The drawing under review shows one solid part. Ordinate dimensions are in mm from its lowest x, y, z. A direction names the side the tool comes from. Round coordinates to 2 decimals unless told otherwise and drop trailing zeros. Order: outer loops, then holes, each group sorted by start corner. A loop starts at its lowest first (then second) coordinate and runs counter-clockwise, first axis right, second up. Notation, with made-up numbers: M -14.5,3.25 L 41.5,3.25 A25 ccw 41.5,39.25 Z; hole C 32.25,-37 d11. An arc over 180 degrees is marked long. Answer as a JSON object with one key per item and string values.
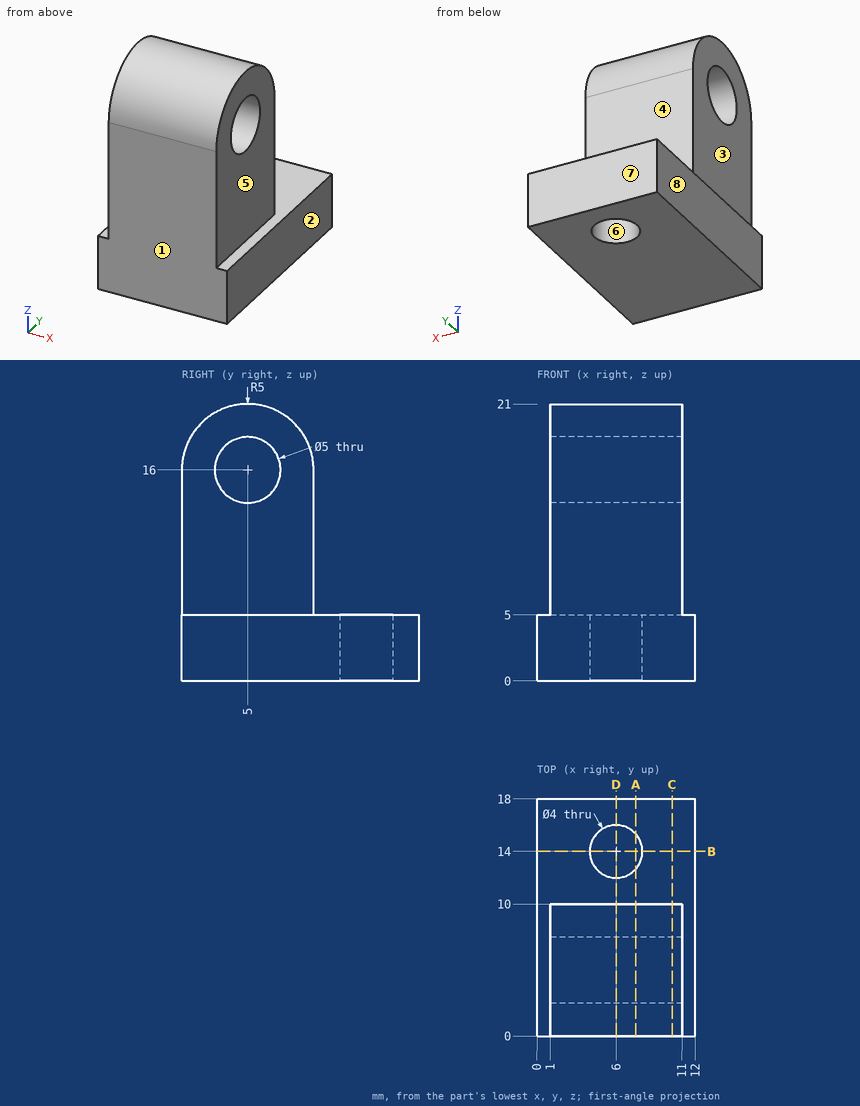
1) Add section D-D on x = 6. State the section outline as (y, z) points, and give its area (3 significant figures).
Geometry check:
{"outline": "M 0,0 L 12,0 L 12,5 L 10,5 L 10,16 A5 ccw 0,16 Z; M 16,0 L 18,0 L 18,5 L 16,5 Z; hole C 5,16 d5", "area": "200 mm²"}
2) Insertion check: P1, Ø3, axis at y = 6.5, z = 18.5, coming from the +X side; P2, Ø3, axis at y = 5.5, z = 14.5, coming from the -X side. Each pin has a flat end and moves straight along its axis. Give the tip position at first contact, or say it passes through.
Geometry check:
{"P1": "stops at x = 11", "P2": "stops at x = 1"}
3) Add section A-A on x = 7.5. State the section outline as (y, z) points, and give its area (3 significant figures).
Geometry check:
{"outline": "M 0,0 L 12.68,0 L 12.68,5 L 10,5 L 10,16 A5 ccw 0,16 Z; M 15.32,0 L 18,0 L 18,5 L 15.32,5 Z; hole C 5,16 d5", "area": "206 mm²"}
4) For L1, parallel to Z at x = 6.75, y = 5; L2, parallel to Y at x = 2.25, z = 6.25; L3, parallel to X at y = 4.5, z = 8, list the stretches that pass through material, from the lowest coordinate up.
Geometry check:
{"L1": "z = 0 to 13.5, 18.5 to 21", "L2": "y = 0 to 10", "L3": "x = 1 to 11"}
5) Add section C-C on x = 10.25. State the section outline as (y, z) points, and give its area (3 significant figures).
Geometry check:
{"outline": "M 0,0 L 18,0 L 18,5 L 10,5 L 10,16 A5 ccw 0,16 Z; hole C 5,16 d5", "area": "220 mm²"}
6) Machinability: for the marked faces 1, 2, 3, 4 and 5, which of the approach directions +Z, -Z, +X, -X, +Y, -Y give a long, thin tool a straight path to every point of the face, cutting with its end or side? Answer none if there is none.
Geometry check:
{"face 1": "+Z, -Z, +X, -X, -Y", "face 2": "+Z, -Z, +X, +Y, -Y", "face 3": "+Z, -X, +Y, -Y", "face 4": "+Z, +X, -X, +Y", "face 5": "+Z, +X, +Y, -Y"}
7) Mouldability with a two-part tool opening along Y and no side actions: class the marked faces 6, 7 and 8 as +Y half, -Y half, draft (parallel to the pull), parting line (faces both ways), or undercut.
Geometry check:
{"face 6": "undercut", "face 7": "+Y half", "face 8": "draft"}
8) Add section B-B on y = 14. State the section outline as (x, z) points.
Geometry check:
{"outline": "M 0,0 L 4,0 L 4,5 L 0,5 Z; M 8,0 L 12,0 L 12,5 L 8,5 Z"}
